Geometry: final body of the model. Coordinates: model frame, mm. Give positions to 0.01 mm unless a question says otherwise; leave off trailing zeros. Loops run counter-clockwise (first coordinate to the right, second up) from the corner with the lowest first, then second, coordinate; pieces in that order, holes last. Notation, with made-up numbers: (68, 45.25) - (102, 45.25) arc R19 ccw to (102, 81.25) - close; hole circle Ø4 at (48, -0.75). An arc over 180 degrees is marked (long way). Use CSV: the item, a comma, the result in double quotes. Start each with the question number.
```python
from build123d import *

# Parameters (mm, degrees)
EXTRUDE_1_DEPTH     = 3
SKETCH_2_R          = 7
CUT_EXTRUDE_1_DEPTH = 80.252760204
SKETCH_3_R          = 1.5
CUT_EXTRUDE_2_DEPTH = 80.252760204
SKETCH_4_R          = 1.5
CUT_EXTRUDE_3_DEPTH = 80.252760204
CHAMFER_1_SIZE      = 2.6


with BuildPart() as part:
    # Эскиз1 → Бобышка-Вытянуть1 (new body)
    with BuildSketch(Plane.XY):
        with BuildLine():
            Line((8, 0), (48, 0))
            ThreePointArc((48, 0), (53.656854249, 2.343145751), (56, 8))
            Line((56, 8), (56, 48))
            ThreePointArc((56, 48), (53.656854249, 53.656854249), (48, 56))
            Line((48, 56), (8, 56))
            ThreePointArc((8, 56), (2.343145751, 53.656854249), (0, 48))
            Line((0, 48), (0, 8))
            ThreePointArc((0, 8), (2.343145751, 2.343145751), (8, 0))
        make_face()
    extrude(amount=EXTRUDE_1_DEPTH)

    # Эскиз2 → Вырез-Вытянуть1 (cut, through all)
    with BuildSketch(Plane.XY.offset(3)):
        with Locations((28, 28)):
            Circle(SKETCH_2_R)
    extrude(amount=-CUT_EXTRUDE_1_DEPTH, mode=Mode.SUBTRACT)

    # Эскиз3 → Вырез-Вытянуть2 (cut, through all)
    with BuildSketch(Plane.XY.offset(3)):
        with Locations((2.67, 12)):
            Circle(SKETCH_3_R)
        with Locations((53.33, 12)):
            Circle(SKETCH_3_R)
        with Locations((53.33, 44)):
            Circle(SKETCH_3_R)
        with Locations((2.67, 44)):
            Circle(SKETCH_3_R)
    extrude(amount=-CUT_EXTRUDE_2_DEPTH, mode=Mode.SUBTRACT)

    # Эскиз4 → Вырез-Вытянуть3 (cut, through all)
    with BuildSketch(Plane.XY.offset(3)):
        with Locations((17, 8)):
            Circle(SKETCH_4_R)
        with Locations((39, 8)):
            Circle(SKETCH_4_R)
        with Locations((39, 48)):
            Circle(SKETCH_4_R)
        with Locations((17, 48)):
            Circle(SKETCH_4_R)
    extrude(amount=-CUT_EXTRUDE_3_DEPTH, mode=Mode.SUBTRACT)

    # Фаска1
    chamfer_1_edges = [part.edges().sort_by_distance(p)[0] for p in [
        (15.5, 48, 3),
        (37.5, 48, 3),
        (37.5, 8, 3),
        (15.5, 8, 3),
    ]]
    chamfer(chamfer_1_edges, length=CHAMFER_1_SIZE)


solid = part.part
```
Item 1: Ray query, probe 1 along Y at (x, z) = (39, 0.25); probe 2 along Y at (x, z) = (28, 2.3); probe 3 along Y at (x, z) = (22.5, 1.9). Return the intervals inside material, ascending.
Item 2: Section C-C (x = 28). Output: boundary loops of the cut face in (y, z), plus the area to 3 significant figures.
Item 3: Section B-B (z = 1.8). Give the number of separate pieces and of enclosed holes in the cut face, plus the area to 3 significant figures.
Item 4: Mould query, pull axis X, two halves, no side actions, for faces 1 (the flat face through (21, 22, 0)), 2 (the cylindrical face through (16.675, 46.536, 0.203)), 3 (the cylindrical face through (2.281, 2.406, 1.479)). Classes: pulls with the +X half, pulls with the -X half, needs draft (parallel to the pull), parting line crosses it, or undercut.
Item 5: Section D-D (x = 53.33). Output: boundary loops of the cut face in (y, z), plus the area to 3 significant figures.
Item 6: Section A-A (x = 17). Output: boundary loops of the cut face in (y, z).
Item 7: Pin query (flat end, axial travel): pin 1 Ø6 at (x, y) = (15.5, 33) entering from -Z; pin 2 Ø2.5 at (x, y) = (17, 8) entering from -Z; pin 3 Ø3.5 at (x, y) = (39, 8) entering from +Z. Return the tip coordinate at first contact, or that it passes through.
Outcome:
1,probe 1,"y = 0 to 6.5, 9.5 to 46.5, 49.5 to 56"
1,probe 2,"y = 0 to 21, 35 to 56"
1,probe 3,"y = 0 to 23.67, 32.33 to 56"
2,outline,"(0, 0) - (21, 0) - (21, 3) - (0, 3) - close; (35, 0) - (56, 0) - (56, 3) - (35, 3) - close"
2,area,"126 mm2"
3,separate pieces,"1"
3,enclosed holes,"9"
3,area,"2,790 mm2"
4,face 1,"needs draft"
4,face 2,"undercut"
4,face 3,"pulls with the -X half"
5,outline,"(2.03, 0) - (10.5, 0) - (10.5, 3) - (2.03, 3) - close; (13.5, 0) - (42.5, 0) - (42.5, 3) - (13.5, 3) - close; (45.5, 0) - (53.97, 0) - (53.97, 3) - (45.5, 3) - close"
5,area,"138 mm2"
6,outline,"(0, 0) - (6.5, 0) - (6.5, 0.4) - (3.9, 3) - (0, 3) - close; (9.5, 0) - (46.5, 0) - (46.5, 0.4) - (43.9, 3) - (12.1, 3) - (9.5, 0.4) - close; (49.5, 0) - (56, 0) - (56, 3) - (52.1, 3) - (49.5, 0.4) - close"
7,pin 1,"stops at z = 0"
7,pin 2,"passes through"
7,pin 3,"stops at z = 0.65"
